Autodesk Inventor part; units mm, degrees
ref_plane "YZ Plane" through (0, 0, 0) normal (1, 0, 0) x (0, 1, 0)
ref_plane "XZ Plane" through (0, 0, 0) normal (0, 1, 0) x (-1, 0, 0)
ref_plane "XY Plane" through (0, 0, 0) normal (0, 0, 1) x (1, 0, 0)
sketch "Sketch1" plane through (0, 0, 0) normal (1, 0, 0) x (0, 1, 0)
  line L0 (9.0511, -31.5552) -> (23.3, -16.54)
  line L1 (23.3, -16.54) -> (23.3033, -19.3531)
  line L2 (10.3088, -33.0443) -> (23.3033, -19.3531)
  arc A0 (9.0511, -31.5552) -> (10.3088, -33.0443) centre (56.5754, 7.3116) ccw
  line L3 (9.674, -32.3047) -> (23.3017, -17.9466)
  line L4 (0, 0) -> (23.3, 0)
  line L5 (0, 0) -> (25.6397, 0)
  line L6 (23.3, 0) -> (23.3, -16.54)
  line L7 (23.3, -16.54) -> (15.899, -24.339)
  line L8 (23.3033, -19.3531) -> (25.6397, -16.8915)
  line L9 (23.3, 0) -> (24.3897, 0)
  line L10 (24.3897, 0) -> (24.3897, -16.8)
  line L11 (23.3017, -17.9466) -> (24.3897, -16.8)
  line L12 (25.6397, 0) -> (25.6397, -16.8915)
  line L13 (25.6397, 0) -> (28.254, 0)
  line L14 (28.254, 0) -> (28.254, -15.1793)
  line L15 (28.254, -15.1793) -> (10.9078, -33.6064)
  arc A1 (10.3088, -33.0443) -> (10.9078, -33.6064) centre (31.8453, -10.6914) ccw
  arc A2 (9.674, -32.3047) -> (10.9976, -33.511) centre (15.0193, -27.7689) ccw
  dimension "d0" = 23.3
  dimension "d1" = 16.54
  dimension "d2" = 18.8761
  dimension "d3" = 20.7
  dimension "d4" = 61.3938
  dimension "d5" = 2.8131
  dimension "d6" = 136.5
  dimension "d18" = 16.8
  dimension "d19" = 1.25
  dimension "d22" = 0.9746
  dimension "d25" = 1.9491
revolve "Revolution1" add sketch "Sketch1" angle 360 about axis through (0, 0, 0) along (0, 1, 0) contours L3 L1 L2 A2 | L11 L10 L5 L12 L8 L1 | L2 L8 L12 L13 L14 L15 A2
sketch "Sketch3" plane through (0, 28.254, 0) normal (0, 1, 0) x (1, 0, 0)
  point P0 (0, 0)
hole "Hole2" at (0, 28.254, 0) direction (0, -1, 0) diameter 12.5 end through all
sketch "Sketch4" plane through (0, 28.254, 0) normal (0, 1, 0) x (1, 0, 0)
  line L0 (-5.9666, 8.9326) -> (-7.9148, 10.5784)
  line L1 (-7.9148, 10.5784) -> (-10.9871, 6.9417)
  line L2 (-10.9871, 6.9417) -> (-9.0388, 5.2958)
  line L3 (-9.0388, 5.2958) -> (-5.9666, 8.9326)
  line L4 (-6.9417, -10.9871) -> (-5.2958, -9.0388)
  line L5 (-8.9326, -5.9666) -> (-10.5784, -7.9148)
  line L6 (-10.5784, -7.9148) -> (-6.9417, -10.9871)
  line L7 (-5.2958, -9.0388) -> (-8.9326, -5.9666)
  line L8 (10.9871, -6.9417) -> (9.0388, -5.2958)
  line L9 (5.9666, -8.9326) -> (7.9148, -10.5784)
  line L10 (7.9148, -10.5784) -> (10.9871, -6.9417)
  line L11 (9.0388, -5.2958) -> (5.9666, -8.9326)
  line L12 (6.9417, 10.9871) -> (5.2958, 9.0388)
  line L13 (8.9326, 5.9666) -> (10.5784, 7.9148)
  line L14 (10.5784, 7.9148) -> (6.9417, 10.9871)
  line L15 (5.2958, 9.0388) -> (8.9326, 5.9666)
  point P0 (0, 0)
  point P1 (-10.0129, 6.1188)
  point P2 (-6.1188, -10.0129)
  point P3 (10.0129, -6.1188)
  point P4 (6.1188, 10.0129)
  dimension "d33" = 4.7607
  dimension "d34" = 2.5504
  dimension "d35" = 5.2958
  dimension "d36" = 9.0388
  dimension "d37" = 6.1188
  dimension "d40" = 360
extrude "Extrusion1" cut sketch "Sketch4" against normal blind 0.5
properties part number "Back Cover"
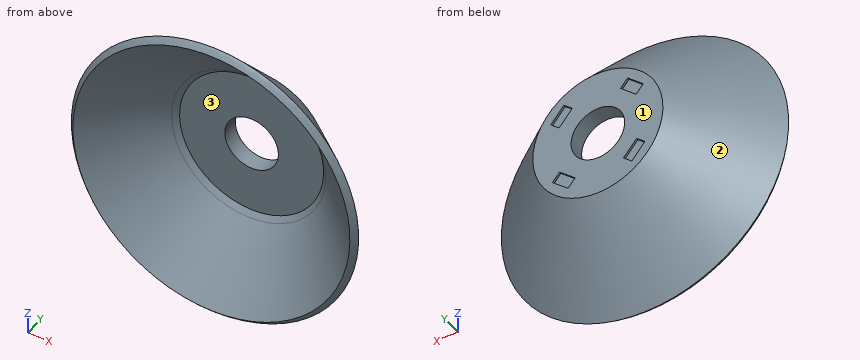
Geometry: final body of the model. Coordinates: model frame, mm. Face numbers are marked on the shaded views. Round coordinates to 2 decimals unless told otherwise and drop trailing zeros. Order: outer loops, then holes, each group sorted by start corner. A loop starts at its lowest first (then second) coordinate and runs counter-clockwise, first axis right, second up. Notation, with made-up numbers: (85, 81) - (118, 81) arc R28 ccw to (118, 111) - close; hole circle Ø7 at (25.25, -5.75). An arc over 180 degrees is marked (long way). Write item = value, one per line. Start each with the question number.
Q1. Pull-direction query (Z, two-part tool) for the marked faces 1, 2 and 3; classes: +Z half, -Z half, draft (parallel to the pull), parting line (faces both ways), or undercut.
Q2. Pin query (flat end, axial travel): pin 1 (4 mm diameter, centred on x = 18, z = 9.5, fed in from +Y); pin 2 (5 mm diameter, centred on x = 15.5, z = 26, fed in from +Y); pin 3 (1 mm diameter, centred on x = -1, z = 19, fed in from +Y). Return the tip coordinate at first contact, or that it passes through.
Q3. Cut plane A-A on z = 0. Return the cut outline in (x, y), and give its area (3 significant figures).
Q4. Ray query, line 1 (Z direction, x = 14.5, y = 22.5); line 2 (X direction, y = 19.5, z = -17); line 3 (Y direction, x = 9, z = 6.5). Return the intervals inside material, ascending. Write a range as from..to.
Q5. Cut plane C-C on y = 13. Return the cut outline in (x, z).
Q6. Cut plane B-B on x = 0. Return the cut outline in (y, z), and give its area (3 significant figures).
Outcome:
q1.face_1 = draft
q1.face_2 = parting line
q1.face_3 = undercut
q2.pin_1 = 25.27
q2.pin_2 = 16.4
q2.pin_3 = 25.1
q3.outline = (-33.51, 11) arc R7.01 ccw to (-32.3, 9.67) - (-17.95, 23.3) - (-16.8, 24.39) - (-6.25, 24.39) - (-6.25, 28.25) - (-15.18, 28.25) - close; (6.25, 24.39) - (16.8, 24.39) - (17.95, 23.3) - (32.3, 9.67) arc R7.01 ccw to (33.51, 11) - (15.18, 28.25) - (6.25, 28.25) - close
q3.area = 157 mm^2
q4.line_1 = -15.59..-11.95, 11.95..15.59
q4.line_2 = -17.61..-13.89, 13.89..17.61
q4.line_3 = 24.39..27.75
q5.outline = circle Ø62.77 at (0, 0); hole circle Ø57.6 at (0, 0)
q6.outline = (9.67, -32.3) arc R7.01 ccw to (11, -33.51) - (28.25, -15.18) - (28.25, -6.25) - (24.39, -6.25) - (24.39, -16.8) - (23.3, -17.95) - close; (9.67, 32.3) - (23.3, 17.95) - (24.39, 16.8) - (24.39, 6.25) - (28.25, 6.25) - (28.25, 15.18) - (11, 33.51) arc R7.01 ccw to start
q6.area = 157 mm^2
